Work out the finished part from the listing and answer in its coordinate system (mm). Face numbers are marked on the shaded views. A direction names the side the tool comes from. Coordinates: 2 decimals unless noted, no trailing zeros. Order: outer loops, then holes, each group sorted by start corner. A loop starts at its lowest first (then second) coordinate and runs counter-clockwise, first axis right, second up. Notation, with made-up numbers: M 26,-37 L 54,-37 A17 ccw 54,-27 Z; hole C -5,-29.75 d1. An arc over 180 degrees is marked long. Use a Markdown table: item, result.
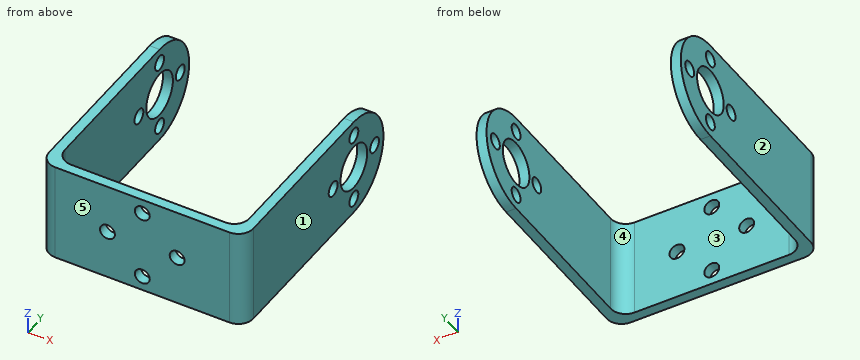
from build123d import *

# Parameters (mm, degrees)
EXTRUDE_1_DEPTH     = 2
SKETCH_2_W          = 2
SKETCH_2_H          = 20
EXTRUDE_2_DEPTH     = 60
FILLET_1_R          = 3
SKETCH_6_R          = 4.5
SKETCH_6_R_2        = 1.5
CUT_EXTRUDE_2_DEPTH = 76
SKETCH_7_R          = 1.5
CUT_EXTRUDE_3_DEPTH = 10


with BuildPart() as part:
    # 草图1 → 凸台-拉伸1 (new body)
    with BuildSketch(Plane(origin=(0, 0, 0), x_dir=(1, 0, 0), z_dir=(0, 1, 0))):
        Polygon((-20.5, 10), (-12.5, 10), (12.5, 10), (20.5, 10), (20.5, -10), (12.5, -10), (-12.5, -10), (-20.5, -10), align=None)
    extrude(amount=EXTRUDE_1_DEPTH)

    # 草图2 → 凸台-拉伸2 (add)
    with BuildSketch(Plane(origin=(0, 2, 0), x_dir=(1, 0, 0), z_dir=(0, 1, 0))):
        with Locations((-19.5, 0)):
            Rectangle(SKETCH_2_W, SKETCH_2_H)
        with Locations((19.5, 0)):
            Rectangle(SKETCH_2_W, SKETCH_2_H)
    extrude(amount=EXTRUDE_2_DEPTH)

    # 圆角1
    fillet_1_edges = [part.edges().sort_by_distance(p)[0] for p in [
        (20.5, 0, 0),
        (-18.5, 2, 0),
        (18.5, 2, 0),
        (-20.5, 0, 0),
    ]]
    fillet(fillet_1_edges, radius=FILLET_1_R)

    # 草图6 → 切除-拉伸2 (cut, through all)
    with BuildSketch(Plane.ZY.offset(20.5)):
        with Locations((0, 37)):
            Circle(SKETCH_6_R)
        with Locations((0, 30)):
            Circle(SKETCH_6_R_2)
        with Locations((-7, 37)):
            Circle(SKETCH_6_R_2)
        with Locations((0, 44)):
            Circle(SKETCH_6_R_2)
        with Locations((7, 37)):
            Circle(SKETCH_6_R_2)
        with BuildLine():
            Line((-10, 37), (-10, 62))
            Line((-10, 62), (10, 62))
            Line((10, 62), (10, 37))
            ThreePointArc((10, 37), (0, 47), (-10, 37))
        make_face()
    extrude(amount=-CUT_EXTRUDE_2_DEPTH, mode=Mode.SUBTRACT)

    # 草图7 → 切除-拉伸3 (cut)
    with BuildSketch(Plane.XZ):
        with Locations(Location((-7, 0, 0), (0, 0, 270))):
            Circle(SKETCH_7_R)
        with Locations(Location((0, 7, 0), (0, 0, 270))):
            Circle(SKETCH_7_R)
        with Locations(Location((7, 0, 0), (0, 0, 270))):
            Circle(SKETCH_7_R)
        with Locations(Location((0, -7, 0), (0, 0, 270))):
            Circle(SKETCH_7_R)
    extrude(amount=-CUT_EXTRUDE_3_DEPTH, mode=Mode.SUBTRACT)


solid = part.part
1. Section A-A on x = 7 is taken. Determine the outline of the cut face in (y, z).
Answers below:
| item | result |
|---|---|
| outline | M 0,-10 L 2,-10 L 2,-1.5 L 0,-1.5 Z; M 0,1.5 L 2,1.5 L 2,10 L 0,10 Z |
2. Section B-B on y = 16.5 is taken. Determine the outline of the cut face in (x, z).
Answers below:
| item | result |
|---|---|
| outline | M -20.5,-10 L -18.5,-10 L -18.5,10 L -20.5,10 Z; M 18.5,-10 L 20.5,-10 L 20.5,10 L 18.5,10 Z |
3. For a pull along X with two mould halves and no side action, classify the marked faces 1, 2 and 3 as +X half, -X half, draft (parallel to the pull), parting line (faces both ways), or undercut.
Answers below:
| item | result |
|---|---|
| face 1 | +X half |
| face 2 | -X half |
| face 3 | undercut |
4. Section C-C on z = 7 is taken. Determine the outline of the cut face in (x, y).
Answers below:
| item | result |
|---|---|
| outline | M -20.5,3 A3 ccw -17.5,0 L -1.5,0 L -1.5,2 L -15.5,2 A3 cw -18.5,5 L -18.5,35.5 L -20.5,35.5 Z; M -20.5,38.5 L -18.5,38.5 L -18.5,44.14 L -20.5,44.14 Z; M 1.5,0 L 17.5,0 A3 ccw 20.5,3 L 20.5,35.5 L 18.5,35.5 L 18.5,5 A3 cw 15.5,2 L 1.5,2 Z; M 18.5,38.5 L 20.5,38.5 L 20.5,44.14 L 18.5,44.14 Z |
5. Flat-ended cylindrical pins translate along their axes: P1, Ø3, axis at x = 12.5, z = -2.5, coming from the +Y side; P2, Ø8, axis at x = -13, z = 5.5, coming from the +Y side. Find the tip coordinate at first contact, or state that the pin passes through.
Answers below:
| item | result |
|---|---|
| P1 | y = 2 |
| P2 | y = 2.4 |
6. Section D-D on y = 30 is taken. Determine the outline of the cut face in (x, z).
Answers below:
| item | result |
|---|---|
| outline | M -20.5,-10 L -18.5,-10 L -18.5,-1.5 L -20.5,-1.5 Z; M -20.5,1.5 L -18.5,1.5 L -18.5,10 L -20.5,10 Z; M 18.5,-10 L 20.5,-10 L 20.5,-1.5 L 18.5,-1.5 Z; M 18.5,1.5 L 20.5,1.5 L 20.5,10 L 18.5,10 Z |
7. Find the intervals of material crossed by probe 1 along X at (y, z) = (30, 3.5); probe 2 along Y at (x, z) = (2, -8.5); probe 3 along Y at (x, z) = (19.9, 7), in increasing order.
Answers below:
| item | result |
|---|---|
| probe 1 | -20.5 to -18.5, 18.5 to 20.5 |
| probe 2 | 0 to 2 |
| probe 3 | 1.2 to 35.5, 38.5 to 44.14 |
8. For the marked faces 4 and 5, determine the directions among +Z, -Z, +X, -X, +Y, -Y from which every point of the face is accessible in a straight line to the end or side of a thin tool.
Answers below:
| item | result |
|---|---|
| face 4 | +Z, -Z, +Y |
| face 5 | +Z, -Z, +X, -X, -Y |
